Work out the finished part from the listing and answer in its coordinate system (mm). A direction names the side the tool comes from. Round coordinates to 2 decimals unless told otherwise and drop trailing zeros. Write each loop counter-clockwise with the first axis right and the second up, starting at its lowest first coordinate (ties: lowest second). Pieces come first, ordered by that corner, then holes. Notation, with made-up numbers: M 7,53 L 33,53 A22 ccw 33,75 Z; hole C -29.75,-33 d11. An arc over 180 degrees is marked long. One line per item, written item: value. Start each with the question number.
Q1. Find section C-C (x = 2.75). Write down the section's boundary in (y, z) (3 decimals), and give its area (3 significant figures).
Q2. Find section D-D (z = -5). Write down the section's boundary in (x, y).
Q3. Consider probe 1 along Y at (x, z) = (-3.75, 0); probe 2 along Z at (x, y) = (-4.9, -11.43) (3 decimals); probe 3 along X at (y, z) = (-5.75, -1.25). Determine where each line is inside the solid, lowest interval first.
Q4. The mould has two halves that part along X. Classify faces 1 (the flat face through (-2, -15, 5.197)), 2 (the flat face through (-4, -6, 9.525)), 3 (the flat face through (-0.526, 6.944, -0.133)): released by +X, released by -X, zero draft, split by the parting line, or undercut.
Q5. Find section A-A (y = -11.43). Write down the section's boundary in (x, z) (3 decimals), and give its area (3 significant figures).
Q6. Given pin 1 Ø5 at (x, z) = (4, 7.5) entering from -Y; pin 2 Ø4.5 at (y, z) = (-11.43, 0) entering from +X; pin 3 Ø8 at (y, z) = (-12, 5) entering from +X, each flat-ended and moving along its own axis, determine where each tip first touches the part or whether it passes through.
Q7. Find section B-B (z = -7.25). Write down the section's boundary in (x, y).
Q8. A tool of negligible diameter and unlimited length cuts with its end or side. For faces 4 (the flat face through (-4.57, -14.68, 3.7)), 5 (the conical face through (-1.945, -9.58, 0.243)), from which of +Z, -Z, +X, -X, +Y, -Y can it reach the whole face along a straight path? Write none if from no direction.
Autodesk Inventor part; units mm, degrees
ref_plane "YZ Plane" through (0, 0, 0) normal (1, 0, 0) x (0, 1, 0)
ref_plane "XZ Plane" through (0, 0, 0) normal (0, 1, 0) x (-1, 0, 0)
ref_plane "XY Plane" through (0, 0, 0) normal (0, 0, 1) x (1, 0, 0)
sketch "Sketch4" plane through (0, 0, 0) normal (0, 0, 1) x (1, 0, 0)
  arc A0 (-0.0698, 6.3496) -> (6.1152, -1.7109) centre (0, 0) ccw
  arc A1 (-0.9946, 7.5548) -> (7.04, -2.916) centre (0, 0) ccw
  line L0 (0, 0) -> (0, 7.9375) construction
  line L1 (-0.0698, 6.3496) -> (6.1152, -1.7109) construction
  line L2 (-0.0698, 6.3496) -> (-0.9946, 7.5548)
  line L3 (6.1152, -1.7109) -> (7.04, -2.916)
  circle A2 centre (0, 0) radius 6.35
  dimension "d10" = 12.7
  dimension "d11" = 1.27
  dimension "d12" = 37.5
  dimension "d13" = 10.16
extrude "Extrusion3" add sketch "Sketch4" along normal mid plane 19.05 contours A0 L3 A1 L2
sketch "Sketch5" plane through (0, 0, 0) normal (0, 0, 1) x (1, 0, 0)
  arc A0 (-0.9946, 7.5548) -> (7.04, -2.916) centre (0, 0) ccw
  line L0 (-7.62, 0) -> (-7.62, -15.24)
  line L1 (-7.62, -15.24) -> (0, -15.24)
  line L2 (0, -15.24) -> (0, -7.62)
  circle A1 centre (0, 0) radius 7.9375
  dimension "d16" = 7.62
extrude "Extrusion4" add sketch "Sketch5" along normal mid plane 19.05 contours A0 L2 A1 L0 | A1 L2 L1 L0 picked at (-7.3048, -2.4081)
sketch "Sketch6" plane through (0, -15.24, 9.525) normal (1, 0, 0) x (0, 0, -1)
  line L0 (0, 7.62) -> (19.05, 7.62)
  line L1 (19.05, 7.62) -> (19.05, 0)
  line L2 (0, 0) -> (19.05, 0)
  line L3 (0, 0) -> (0, 7.62)
  line L4 (0, 7.62) -> (19.05, 0) construction
  line L5 (19.05, 7.62) -> (0, 0) construction
  point P0 (9.525, 15.24)
  point P1 (9.525, 3.81)
hole "Hole1" at (0, -11.43, 0) direction (-1, 0, 0) diameter 3.5052 end through all countersink diameter 7.112 countersink angle 82
sketch "Sketch10" plane through (-7.62, -15.24, 9.525) normal (0, -1, 0) x (1, 0, 0)
  line L0 (0, -19.05) -> (0, 0)
  line L1 (7.62, -19.05) -> (0, -19.05)
  line L2 (7.62, 0) -> (7.62, -19.05)
  line L3 (0, 0) -> (7.62, 0)
  line L4 (3.81, -19.05) -> (3.81, 0) construction
  spline S0 degree 2 poles (2.8014, -11.7171) (3.1307, -11.7171) (3.7235, -11.9518) (3.9294, -12.1617) knots 0 0 0 1 2 2 2
  spline S1 degree 2 poles (3.9294, -12.1617) (4.1887, -12.4252) (4.4563, -13.1374) (4.4563, -13.6808) knots 0 0 0 1 2 2 2
  line L5 (4.4563, -13.6808) -> (4.4563, -14.253)
  line L6 (4.4563, -14.253) -> (6.35, -14.253)
  line L7 (6.35, -14.253) -> (6.35, -14.9282)
  line L8 (6.35, -14.9282) -> (1.27, -14.9282)
  line L9 (1.27, -14.9282) -> (1.27, -13.652)
  spline S2 degree 2 poles (1.27, -13.652) (1.27, -13.1991) (1.4182, -12.5652) (1.587, -12.3223) knots 0 0 0 1 2 2 2
  spline S3 degree 2 poles (1.587, -12.3223) (1.7805, -12.0382) (2.3774, -11.7171) (2.8014, -11.7171) knots 0 0 0 1 2 2 2
  spline S4 degree 2 poles (2.822, -12.4211) (2.5585, -12.4211) (2.1716, -12.6022) (2.0481, -12.7875) knots 0 0 0 1 2 2 2
  spline S5 degree 2 poles (2.0481, -12.7875) (1.941, -12.948) (1.8546, -13.3762) (1.8546, -13.6932) knots 0 0 0 1 2 2 2
  line L10 (1.8546, -13.6932) -> (1.8546, -14.253)
  line L11 (1.8546, -14.253) -> (3.88, -14.253)
  line L12 (3.88, -14.253) -> (3.88, -13.792)
  spline S6 degree 2 poles (3.88, -13.792) (3.88, -13.3803) (3.7482, -12.8739) (3.5753, -12.7093) knots 0 0 0 1 2 2 2
  spline S7 degree 2 poles (3.5753, -12.7093) (3.423, -12.5569) (3.0649, -12.4211) (2.822, -12.4211) knots 0 0 0 1 2 2 2
  line L13 (1.27, -7.3905) -> (6.35, -9.1401)
  line L14 (6.35, -9.1401) -> (6.35, -9.8687)
  line L15 (6.35, -9.8687) -> (1.27, -11.6183)
  line L16 (1.27, -11.6183) -> (1.27, -10.8938)
  line L17 (1.27, -10.8938) -> (5.4896, -9.4859)
  line L18 (5.4896, -9.4859) -> (1.27, -8.078)
  line L19 (1.27, -8.078) -> (1.27, -7.3905)
  line L20 (4.6045, -3.7225) -> (4.6045, -4.3277)
  line L21 (4.6045, -4.3277) -> (6.35, -4.3277)
  line L22 (6.35, -4.3277) -> (6.35, -4.9822)
  line L23 (6.35, -4.9822) -> (4.6045, -4.9822)
  line L24 (4.6045, -4.9822) -> (4.6045, -7.2258)
  line L25 (4.6045, -7.2258) -> (3.8882, -7.2258)
  line L26 (3.8882, -7.2258) -> (1.27, -4.9534)
  line L27 (1.27, -4.9534) -> (1.27, -4.3277)
  line L28 (1.27, -4.3277) -> (4.057, -4.3277)
  line L29 (4.057, -4.3277) -> (4.057, -3.7225)
  line L30 (4.057, -3.7225) -> (4.6045, -3.7225)
  line L31 (4.057, -4.9822) -> (2.0728, -4.9822)
  line L32 (2.0728, -4.9822) -> (4.057, -6.6907)
  line L33 (4.057, -6.6907) -> (4.057, -4.9822)
  point P0 (7.62, -9.525)
extrude "Text" cut sketch "Sketch10" against normal blind 1.143 contours S0 S1 L5 L6 L7 L8 L9 S2 S3 | L13 L14 L15 L16 L17 L18 L19 | L20 L21 L22 L23 L24 L25 L26 L27 L28 L29 L30
equation "\"d10\" = shadeDiameter"
equation "\"d11\" = shadeHolderWallThickness"
equation "\"d13\" = openingForShade"
equation "\"d14\" = partWidth"
equation "\"d16\" = flatBelowShade"
equation "\"d17\" = partWidth"
equation "\"d28\" = textDepth"
equation "\"shadeDiameter\" = 12.7"
equation "\"partWidth\" = 19.05"
equation "\"backThickness\" = 1.905"
equation "\"backHeight\" = 25.4"
equation "\"cutTiltAngle\" = 52.5deg"
equation "\"flatBelowShade\" = 7.62"
equation "\"shadeHolderWallThickness\" = 1.27"
equation "\"openingForShade\" = 10.16"
equation "\"textDepth\" = 1.143"
properties part number "shadeHolderV02"
The answers:
1. outline: M -7.106,-9.525 L -5.724,-9.525 L -5.724,9.525 L -7.106,9.525 Z
1. area: 26.3 mm2
2. outline: M -7.62,-15.24 L -6.35,-15.24 L -6.35,-14.1 L -1.27,-14.1 L -1.27,-15.24 L 0,-15.24 L 0,-7.62 A7.62 ccw 7.04,-2.92 L 6.12,-1.71 A6.35 cw long -0.07,6.35 L -0.99,7.55 A7.62 ccw -7.62,0 Z
3. probe 1: -15.24 to -13.18, -9.68 to -5.12, 5.12 to 6.63
3. probe 2: -9.525 to -1.753, 1.753 to 9.525
3. probe 3: -7.62 to -2.69, 2.69 to 5
4. face 1: undercut
4. face 2: zero draft
4. face 3: released by +X
5. outline: M -7.62,-9.525 L 0,-9.525 L 0,-3.556 L -2.075,-1.753 L -7.62,-1.753 Z; M -7.62,1.753 L -2.075,1.753 L 0,3.556 L 0,9.525 L -7.62,9.525 Z
5. area: 115 mm2
6. pin 1: y = -7.47
6. pin 2: x = -1.5
6. pin 3: x = 0
7. outline: M -7.62,-15.24 L 0,-15.24 L 0,-7.62 A7.62 ccw 7.04,-2.92 L 6.12,-1.71 A6.35 cw long -0.07,6.35 L -0.99,7.55 A7.62 ccw -7.62,0 Z
8. face 4: -Y
8. face 5: +X
